For this review, take the finished solid that the model builds, in its own axes (mm). A direction names the side the tool comes from. Give positions to 0.01 mm unless a question says otherwise; leave off trailing zeros. Order: outer loops, then holes, each group sorted by start corner. A loop starts at its lowest first (then second) coordinate and runs counter-clockwise, first axis right, second up. Notation, with made-up numbers: (56, 69) -> (95, 69) arc R22 ccw to (95, 102) -> close; hole circle Ø10 at (-26, 82). An arc over 180 degrees is marked (long way). Return JSON: item names as keys, results as strings. Group by question number.
1) To check wall thickness, follow line 1 along Y through (x, z) = (-7, 4); line 2 along X through (y, z) = (15, 8). State the ranges of each line that lie inside material, in increasing order.
2) Add section A-A (y = -8). Give the boundary of the cut face in (x, z), then the cut area to 3 significant figures.
3) Add section D-D (x = 12). Give the boundary of the cut face in (y, z), then the cut area to 3 significant figures.
4) Insertion check: P1, Ø1.8, axis at y = 3, z = 2.5, coming from the -X side. The pin has a flat end and moves straight along its axis. Give the tip position at first contact, or say it passes through.
5) Add section C-C (z = 11.75). Give the boundary of the cut face in (x, y), then the cut area to 3 significant figures.
6) The part is to be moulded in two halves that separate along X. For faces 4 (the face through (0, -15, 0)), 5 (the face through (-13.5, 3.5, 6.1)), 6 (the face through (16.395, 16.332, 7.05)), say which applies: released by +X, released by -X, zero draft, split by the parting line, or undercut.
7) For faces 1 (the face through (-11.5, 2.1, 6.5)), 2 (the face through (13.5, -2, 9)), 3 (the face through (15.5, 2, 5)), list the 3-axis set-ups (+Z, -Z, +X, -X, +Y, -Y) from which the entire face can be reached by the end or side of a thin tool; tool diameter is ignored.
from build123d import *

# Parameters (mm, degrees)
F0_W     = 2
F0_H     = 6.1
F0_H_2   = 2
F0_W_2   = 2.05
F0_H_3   = 5
F1_DEPTH = 14.3
F2_ANGLE = 180
F3_ANGLE = 180


with BuildPart() as f1:
    # F0 (on Top) → F1 (new body)
    with BuildSketch(Plane.XY):
        with BuildLine():
            ThreePointArc((-13.5, 9.45), (-14.5342970466, 9.5842970466), (-15.5, 9.9782816694))
            Line((-15.5, 9.9782816694), (-15.5, 9.45))
            Line((-15.5, 9.45), (-13.5, 9.45))
        make_face()
        with BuildLine():
            ThreePointArc((-9.45, 13.5), (-10.6362175362, 16.3637824638), (-13.5, 17.55))
            ThreePointArc((-13.5, 17.55), (-16.3637824638, 16.3637824638), (-17.55, 13.5))
            ThreePointArc((-17.55, 13.5), (-17.0001785669, 11.4625383439), (-15.5, 9.9782816694))
            Line((-15.5, 9.9782816694), (-15.5, 11.45))
            Line((-15.5, 11.45), (-13.5, 11.45))
            ThreePointArc((-13.5, 11.45), (-14.9495689014, 14.9495689014), (-11.45, 13.5))
            Line((-11.45, 13.5), (-9.45, 13.5))
        make_face()
        with BuildLine():
            Line((-15.5, 11.45), (-15.5, 9.9782816694))
            ThreePointArc((-15.5, 9.9782816694), (-14.5342970466, 9.5842970466), (-13.5, 9.45))
            Line((-13.5, 9.45), (-13.5, 11.45))
            Line((-13.5, 11.45), (-15.5, 11.45))
        make_face()
        with BuildLine():
            ThreePointArc((-15.5, 9.9782816694), (-17.0001785669, 11.4625383439), (-17.55, 13.5))
            Line((-17.55, 13.5), (-17.55, 8.35))
            Line((-17.55, 8.35), (-15.5, 8.35))
            Line((-15.5, 8.35), (-15.5, 9.45))
            Line((-15.5, 9.45), (-15.5, 9.9782816694))
        make_face()
        with Locations((-14.5, 0.3)):
            Rectangle(F0_W, F0_H)
        with Locations((-14.5, -3.75)):
            Rectangle(F0_W, F0_H_2)
        with BuildLine():
            ThreePointArc((-13.5, -9.45), (-16.3637824638, -10.6362175362), (-17.55, -13.5))
            ThreePointArc((-17.55, -13.5), (-16.3637824638, -16.3637824638), (-13.5, -17.55))
            ThreePointArc((-13.5, -17.55), (-10.6362175362, -16.3637824638), (-9.45, -13.5))
            Line((-9.45, -13.5), (-11.45, -13.5))
            ThreePointArc((-11.45, -13.5), (-14.9495689014, -14.9495689014), (-13.5, -11.45))
            Line((-13.5, -11.45), (-13.5, -9.45))
        make_face()
        with BuildLine():
            Line((-13.5, -17.55), (13.5, -17.55))
            ThreePointArc((13.5, -17.55), (10.6362175362, -16.3637824638), (9.45, -13.5))
            Line((9.45, -13.5), (-9.45, -13.5))
            ThreePointArc((-9.45, -13.5), (-10.6362175362, -16.3637824638), (-13.5, -17.55))
        make_face()
        with BuildLine():
            ThreePointArc((-9.45, -13.5), (-10.6362175362, -10.6362175362), (-13.5, -9.45))
            Line((-13.5, -9.45), (-13.5, -11.45))
            ThreePointArc((-13.5, -11.45), (-12.0504310986, -12.0504310986), (-11.45, -13.5))
            Line((-11.45, -13.5), (-9.45, -13.5))
        make_face()
        with BuildLine():
            ThreePointArc((13.5, -17.55), (16.3637824638, -16.3637824638), (17.55, -13.5))
            ThreePointArc((17.55, -13.5), (16.3637824638, -10.6362175362), (13.5, -9.45))
            Line((13.5, -9.45), (13.5, -11.45))
            ThreePointArc((13.5, -11.45), (14.9495689014, -12.0504310986), (15.55, -13.5))
            ThreePointArc((15.55, -13.5), (13.5, -15.55), (11.45, -13.5))
            Line((11.45, -13.5), (9.45, -13.5))
            ThreePointArc((9.45, -13.5), (10.6362175362, -16.3637824638), (13.5, -17.55))
        make_face()
        with BuildLine():
            Line((13.5, -11.45), (13.5, -9.45))
            ThreePointArc((13.5, -9.45), (10.6362175362, -10.6362175362), (9.45, -13.5))
            Line((9.45, -13.5), (11.45, -13.5))
            ThreePointArc((11.45, -13.5), (12.0504310986, -12.0504310986), (13.5, -11.45))
        make_face()
        with BuildLine():
            Line((17.55, 8.35), (17.55, 13.5))
            ThreePointArc((17.55, 13.5), (17.0001785669, 11.4625383439), (15.5, 9.9782816694))
            Line((15.5, 9.9782816694), (15.5, 9.45))
            Line((15.5, 9.45), (15.5, 8.35))
            Line((15.5, 8.35), (17.55, 8.35))
        make_face()
        with Locations((14.5, -3.75)):
            Rectangle(F0_W, F0_H_2)
        with Locations((14.5, 0.3)):
            Rectangle(F0_W, F0_H)
        with BuildLine():
            Line((15.5, 9.45), (15.5, 9.9782816694))
            ThreePointArc((15.5, 9.9782816694), (14.5342970466, 9.5842970466), (13.5, 9.45))
            Line((13.5, 9.45), (15.5, 9.45))
        make_face()
        with BuildLine():
            ThreePointArc((13.5, 9.45), (14.5342970466, 9.5842970466), (15.5, 9.9782816694))
            Line((15.5, 9.9782816694), (15.5, 11.45))
            Line((15.5, 11.45), (13.5, 11.45))
            Line((13.5, 11.45), (13.5, 9.45))
        make_face()
        with BuildLine():
            ThreePointArc((11.5, 9.9782816694), (12.4657029534, 9.5842970466), (13.5, 9.45))
            Line((13.5, 9.45), (13.5, 11.45))
            Line((13.5, 11.45), (11.5, 11.45))
            Line((11.5, 11.45), (11.5, 9.9782816694))
        make_face()
        with BuildLine():
            Line((11.5, 11.45), (10.0071501607, 11.45))
            ThreePointArc((10.0071501607, 11.45), (10.6567028733, 10.6158776986), (11.5, 9.9782816694))
            Line((11.5, 9.9782816694), (11.5, 11.45))
        make_face()
        with BuildLine():
            Line((11.45, 13.5), (9.45, 13.5))
            ThreePointArc((9.45, 13.5), (9.5917688241, 12.4378187182), (10.0071501607, 11.45))
            Line((10.0071501607, 11.45), (11.5, 11.45))
            Line((11.5, 11.45), (13.5, 11.45))
            ThreePointArc((13.5, 11.45), (12.0504310986, 12.0504310986), (11.45, 13.5))
        make_face()
        with BuildLine():
            ThreePointArc((17.55, 13.5), (16.3637824638, 16.3637824638), (13.5, 17.55))
            ThreePointArc((13.5, 17.55), (10.6362175362, 16.3637824638), (9.45, 13.5))
            Line((9.45, 13.5), (11.45, 13.5))
            ThreePointArc((11.45, 13.5), (13.5, 15.55), (15.55, 13.5))
            ThreePointArc((15.55, 13.5), (14.9495689014, 12.0504310986), (13.5, 11.45))
            Line((13.5, 11.45), (15.5, 11.45))
            Line((15.5, 11.45), (15.5, 9.9782816694))
            ThreePointArc((15.5, 9.9782816694), (17.0001785669, 11.4625383439), (17.55, 13.5))
        make_face()
        with BuildLine():
            ThreePointArc((9.45, 13.5), (10.6362175362, 16.3637824638), (13.5, 17.55))
            Line((13.5, 17.55), (-13.5, 17.55))
            ThreePointArc((-13.5, 17.55), (-10.6362175362, 16.3637824638), (-9.45, 13.5))
            Line((-9.45, 13.5), (9.45, 13.5))
        make_face()
        with BuildLine():
            ThreePointArc((-10.0071501607, 11.45), (-9.5917688241, 12.4378187182), (-9.45, 13.5))
            Line((-9.45, 13.5), (-11.45, 13.5))
            ThreePointArc((-11.45, 13.5), (-12.0504310986, 12.0504310986), (-13.5, 11.45))
            Line((-13.5, 11.45), (-11.5, 11.45))
            Line((-11.5, 11.45), (-10.0071501607, 11.45))
        make_face()
        with BuildLine():
            Line((-11.5, 11.45), (-13.5, 11.45))
            Line((-13.5, 11.45), (-13.5, 9.45))
            ThreePointArc((-13.5, 9.45), (-12.4657029534, 9.5842970466), (-11.5, 9.9782816694))
            Line((-11.5, 9.9782816694), (-11.5, 11.45))
        make_face()
        with BuildLine():
            ThreePointArc((-11.5, 9.9782816694), (-10.6567028733, 10.6158776986), (-10.0071501607, 11.45))
            Line((-10.0071501607, 11.45), (-11.5, 11.45))
            Line((-11.5, 11.45), (-11.5, 9.9782816694))
        make_face()
        with BuildLine():
            Line((-15.5, 3.35), (-17.55, 3.35))
            Line((-17.55, 3.35), (-17.55, -13.5))
            ThreePointArc((-17.55, -13.5), (-16.3637824638, -10.6362175362), (-13.5, -9.45))
            Line((-13.5, -9.45), (-13.5, -4.75))
            Line((-13.5, -4.75), (-15.5, -4.75))
            Line((-15.5, -4.75), (-15.5, -2.75))
            Line((-15.5, -2.75), (-15.5, 3.35))
        make_face()
        with Locations((-16.525, 5.85)):
            Rectangle(F0_W_2, F0_H_3)
        Polygon((-15.5, 9.45), (-15.5, 8.35), (-15.5, 3.35), (-13.5, 3.35), (-13.5, 9.45), align=None)
        with Locations((16.525, 5.85)):
            Rectangle(F0_W_2, F0_H_3)
        Polygon((15.5, 3.35), (15.5, 8.35), (15.5, 9.45), (13.5, 9.45), (13.5, 3.35), align=None)
        with BuildLine():
            Line((17.55, -13.5), (17.55, 3.35))
            Line((17.55, 3.35), (15.5, 3.35))
            Line((15.5, 3.35), (15.5, -2.75))
            Line((15.5, -2.75), (15.5, -4.75))
            Line((15.5, -4.75), (13.5, -4.75))
            Line((13.5, -4.75), (13.5, -9.45))
            ThreePointArc((13.5, -9.45), (16.3637824638, -10.6362175362), (17.55, -13.5))
        make_face()
    extrude(amount=F1_DEPTH)

    # F0 (on Top) → F2 (revolve)
    with BuildSketch(Plane.XY):
        with Locations((-16.525, 5.85)):
            Rectangle(F0_W_2, F0_H_3)
        Polygon((-15.5, 9.45), (-15.5, 8.35), (-15.5, 3.35), (-13.5, 3.35), (-13.5, 9.45), align=None)
        with Locations((-12.5, 6.4)):
            Rectangle(F0_W, F0_H)
        with BuildLine():
            Line((-11.5, 11.45), (-13.5, 11.45))
            Line((-13.5, 11.45), (-13.5, 9.45))
            ThreePointArc((-13.5, 9.45), (-12.4657029534, 9.5842970466), (-11.5, 9.9782816694))
            Line((-11.5, 9.9782816694), (-11.5, 11.45))
        make_face()
        with BuildLine():
            Line((-15.5, 11.45), (-15.5, 9.9782816694))
            ThreePointArc((-15.5, 9.9782816694), (-14.5342970466, 9.5842970466), (-13.5, 9.45))
            Line((-13.5, 9.45), (-13.5, 11.45))
            Line((-13.5, 11.45), (-15.5, 11.45))
        make_face()
        with BuildLine():
            ThreePointArc((11.5, 9.9782816694), (12.4657029534, 9.5842970466), (13.5, 9.45))
            Line((13.5, 9.45), (13.5, 11.45))
            Line((13.5, 11.45), (11.5, 11.45))
            Line((11.5, 11.45), (11.5, 9.9782816694))
        make_face()
        with Locations((12.5, 6.4)):
            Rectangle(F0_W, F0_H)
        Polygon((15.5, 3.35), (15.5, 8.35), (15.5, 9.45), (13.5, 9.45), (13.5, 3.35), align=None)
        with BuildLine():
            ThreePointArc((13.5, 9.45), (14.5342970466, 9.5842970466), (15.5, 9.9782816694))
            Line((15.5, 9.9782816694), (15.5, 11.45))
            Line((15.5, 11.45), (13.5, 11.45))
            Line((13.5, 11.45), (13.5, 9.45))
        make_face()
        with Locations((16.525, 5.85)):
            Rectangle(F0_W_2, F0_H_3)
        with BuildLine():
            Line((-11.5, 9.45), (-11.5, 9.9782816694))
            ThreePointArc((-11.5, 9.9782816694), (-12.4657029534, 9.5842970466), (-13.5, 9.45))
            Line((-13.5, 9.45), (-11.5, 9.45))
        make_face()
        with BuildLine():
            ThreePointArc((-13.5, 9.45), (-14.5342970466, 9.5842970466), (-15.5, 9.9782816694))
            Line((-15.5, 9.9782816694), (-15.5, 9.45))
            Line((-15.5, 9.45), (-13.5, 9.45))
        make_face()
        with BuildLine():
            Line((15.5, 9.45), (15.5, 9.9782816694))
            ThreePointArc((15.5, 9.9782816694), (14.5342970466, 9.5842970466), (13.5, 9.45))
            Line((13.5, 9.45), (15.5, 9.45))
        make_face()
        with BuildLine():
            Line((11.5, 9.45), (13.5, 9.45))
            ThreePointArc((13.5, 9.45), (12.4657029534, 9.5842970466), (11.5, 9.9782816694))
            Line((11.5, 9.9782816694), (11.5, 9.45))
        make_face()
    revolve(axis=Axis((0, 3.35, 0), (1, 0, 0)), revolution_arc=F2_ANGLE)

    # F0 (on Top) → F3 (revolve, cut)
    with BuildSketch(Plane.XY):
        Polygon((15.5, 3.35), (15.5, 8.35), (15.5, 9.45), (13.5, 9.45), (13.5, 3.35), align=None)
        with Locations((16.525, 5.85)):
            Rectangle(F0_W_2, F0_H_3)
        with Locations((12.5, 6.4)):
            Rectangle(F0_W, F0_H)
        with Locations((-12.5, 6.4)):
            Rectangle(F0_W, F0_H)
        Polygon((-15.5, 9.45), (-15.5, 8.35), (-15.5, 3.35), (-13.5, 3.35), (-13.5, 9.45), align=None)
        with Locations((-16.525, 5.85)):
            Rectangle(F0_W_2, F0_H_3)
    revolve(axis=Axis((0, 3.35, 0), (1, 0, 0)), revolution_arc=F3_ANGLE, mode=Mode.SUBTRACT)


solid = f1.part
Evaluation:
{
 "1": {"line 1": "-17.55 to -13.5, 13.5 to 17.55", "line 2": "-17.26 to -14.9, -12.1 to 12.1, 14.9 to 17.26"},
 "2": {"outline": "(-17.55, 0) -> (-13.5, 0) -> (-13.5, 14.3) -> (-17.55, 14.3) -> close; (13.5, 0) -> (17.55, 0) -> (17.55, 14.3) -> (13.5, 14.3) -> close", "area": "116 mm^2"},
 "3": {"outline": "(-17.55, 0) -> (-14.9, 0) -> (-14.9, 14.3) -> (-17.55, 14.3) -> close; (-12.1, 0) -> (-9.74, 0) -> (-9.74, 14.3) -> (-12.1, 14.3) -> close; (-4.75, 0) -> (-2.75, 0) arc R6.1 cw to (9.45, 0) -> (12.1, 0) -> (12.1, 14.3) -> (9.74, 14.3) -> (9.74, 4.98) arc R8.1 ccw to start; (14.9, 0) -> (17.55, 0) -> (17.55, 14.3) -> (14.9, 14.3) -> close", "area": "182 mm^2"},
 "4": {"P1": "through"},
 "5": {"outline": "(-17.55, -13.5) arc R4.05 ccw to (-13.5, -17.55) -> (13.5, -17.55) arc R4.05 ccw to (17.55, -13.5) -> (17.55, 13.5) arc R4.05 ccw to (13.5, 17.55) -> (-13.5, 17.55) arc R4.05 ccw to (-17.55, 13.5) -> close; hole circle Ø4.1 at (-13.5, -13.5); hole circle Ø4.1 at (-13.5, 13.5); hole (-13.5, -9.45) arc R4.05 cw to (-9.45, -13.5) -> (9.45, -13.5) arc R4.05 cw to (13.5, -9.45) -> (13.5, 9.45) arc R4.05 cw to (9.45, 13.5) -> (-9.45, 13.5) arc R4.05 cw to (-13.5, 9.45) -> close; hole circle Ø4.1 at (13.5, -13.5); hole circle Ø4.1 at (13.5, 13.5)", "area": "488 mm^2"},
 "6": {"face 4": "zero draft", "face 5": "undercut", "face 6": "released by +X"},
 "7": {"face 1": "+Z, -Z", "face 2": "+Z", "face 3": "-Z"}
}
